Read the model definition and answer for the solid it produces. Units are mm, in the model's axes. A direction names the side the tool comes from. Coordinates: 2 decimals unless noted, no trailing zeros. Loops run counter-clockwise (first coordinate to the right, second up) from the corner with the lowest first, then second, coordinate; pieces in that order, holes last. Notation, with made-up numbers: (78, 64.25) - (124, 64.25) arc R17 cw to (124, 82.25) - close; hole circle Ø5 at (12, 61.25). An arc over 180 degrees is marked (long way). Use one line per item in the form item = value.
from build123d import *

# Parameters (mm, degrees)
SKETCH1_W                      = 75
SKETCH1_H                      = 54.33
BOSS_EXTRUDE1_DEPTH            = 45
CBORE_FOR_M4_SHCS1_D           = 4.5
CBORE_FOR_M4_SHCS1_CBORE_D     = 8
CBORE_FOR_M4_SHCS1_CBORE_DEPTH = 4
SKETCH4_OUTSIDE_W              = 97.592
SKETCH4_OUTSIDE_H              = 67.592
SKETCH4_OUTSIDE_W_2            = 75
SKETCH4_OUTSIDE_H_2            = 40
CUT_EXTRUDE1_DEPTH             = 55.33
SKETCH5_R                      = 8.5
CUT_EXTRUDE2_DEPTH             = 30
SKETCH5_3_R                    = 9
CUT_EXTRUDE3_DEPTH             = 20
SKETCH5_4_R                    = 11
CUT_EXTRUDE4_DEPTH             = 17
SKETCH6_R                      = 3.5
CUT_EXTRUDE5_DEPTH             = 55.33
SKETCH29_OUTSIDE_W             = 97.176
SKETCH29_OUTSIDE_H             = 76.506
SKETCH29_OUTSIDE_R             = 27.165
CUT_EXTRUDE6_DEPTH             = 34
SKETCH30_R                     = 4.5
CUT_EXTRUDE7_DEPTH             = 5


with BuildPart() as part:
    # Sketch1 → Boss-Extrude1 (new body)
    with BuildSketch(Plane.XY):
        Rectangle(SKETCH1_W, SKETCH1_H)
    extrude(amount=BOSS_EXTRUDE1_DEPTH)

    # CBORE for M4 SHCS1 (through all)
    with Locations(Plane.XY.offset(45)):
        with Locations((26.685, -23.265), (26.685, 23.265), (-26.685, 23.265), (-26.685, -23.265)):
            CounterBoreHole(CBORE_FOR_M4_SHCS1_D / 2, CBORE_FOR_M4_SHCS1_CBORE_D / 2, CBORE_FOR_M4_SHCS1_CBORE_DEPTH)

    # Sketch4 outside → Cut-Extrude1 (cut, through all)
    with BuildSketch(Plane.XZ.offset(27.165)):
        with Locations((0, 22.5)):
            Rectangle(SKETCH4_OUTSIDE_W, SKETCH4_OUTSIDE_H)
        with Locations((0, 20)):
            Rectangle(SKETCH4_OUTSIDE_W_2, SKETCH4_OUTSIDE_H_2, mode=Mode.SUBTRACT)
    extrude(amount=-CUT_EXTRUDE1_DEPTH, mode=Mode.SUBTRACT)

    # Sketch5 → Cut-Extrude2 (cut)
    with BuildSketch(Plane.XY.offset(40)):
        Circle(SKETCH5_R)
    extrude(amount=-CUT_EXTRUDE2_DEPTH, mode=Mode.SUBTRACT)

    # Sketch5<3> → Cut-Extrude3 (cut)
    with BuildSketch(Plane.XY.offset(40)):
        Circle(SKETCH5_3_R)
    extrude(amount=-CUT_EXTRUDE3_DEPTH, mode=Mode.SUBTRACT)

    # Sketch5<4> → Cut-Extrude4 (cut)
    with BuildSketch(Plane.XY.offset(40)):
        Circle(SKETCH5_4_R)
    extrude(amount=-CUT_EXTRUDE4_DEPTH, mode=Mode.SUBTRACT)

    # Sketch6 → Cut-Extrude5 (cut, through all)
    with BuildSketch(Plane(origin=(0, 27.165, 0), x_dir=(1, 0, 0), z_dir=(0, 1, 0))):
        with Locations((0, -30)):
            Circle(SKETCH6_R)
    extrude(amount=-CUT_EXTRUDE5_DEPTH, mode=Mode.SUBTRACT)

    # Sketch29 outside → Cut-Extrude6 (cut)
    with BuildSketch(Plane.XY.offset(40)):
        Rectangle(SKETCH29_OUTSIDE_W, SKETCH29_OUTSIDE_H)
        Circle(SKETCH29_OUTSIDE_R, mode=Mode.SUBTRACT)
    extrude(amount=-CUT_EXTRUDE6_DEPTH, mode=Mode.SUBTRACT)

    # Sketch30 → Cut-Extrude7 (cut)
    with BuildSketch(Plane(origin=(0, 0, 0), x_dir=(-1, 0, 0), z_dir=(0, 0, -1))):
        with Locations((-13.555, 11.3)):
            Circle(SKETCH30_R)
        with Locations((13.555, 11.3)):
            Circle(SKETCH30_R)
        with Locations((13.555, -11.3)):
            Circle(SKETCH30_R)
        with Locations((-13.555, -11.3)):
            Circle(SKETCH30_R)
    extrude(amount=-CUT_EXTRUDE7_DEPTH, mode=Mode.SUBTRACT)


solid = part.part
Item 1: Each of these flat-tipped pins is pushed along its axis until it touches: P1, Ø8, axis at x = -6.5, z = 26, coming from the -Y side; P2, Ø5, axis at x = -26.685, y = -23.265, coming from the +Z side; P3, Ø5, axis at y = 19, z = 33.5, coming from the -X side. Where does it stop, or does it pass through?
Results below:
P1 = -27.05
P2 = 6
P3 = -21.58
Item 2: Which of the six approach directions +Z, -Z, +X, -X, +Y, -Y give full straight-line access (tool end or side, diameter ignored) to faces 1 (the flat face through (37.5, 0, 3)), 2 (the flat face through (-27.35, 0.38, 6)), 3 (the flat face through (14, -11, 5)), 4 (the flat face through (0, 0, 10)), 5 (the flat face through (12, 0, 40))?
Results below:
face_1 = +Z, -Z, +X, +Y, -Y
face_2 = +Z, -X
face_3 = -Z
face_4 = +Z
face_5 = +Z, +X, -X, +Y, -Y
Item 3: The part is cut by section B-B on y = 0. Give the vertices of the cut face in (x, z) (3 decimals).
Results below:
outline = (-37.5, 0) - (37.5, 0) - (37.5, 6) - (27.165, 6) - (27.165, 40) - (11, 40) - (11, 23) - (9, 23) - (9, 20) - (8.5, 20) - (8.5, 10) - (-8.5, 10) - (-8.5, 20) - (-9, 20) - (-9, 23) - (-11, 23) - (-11, 40) - (-27.165, 40) - (-27.165, 6) - (-37.5, 6) - close
Item 4: For a pull along Z with two mould halves and no side action, classify faces 6 (the cylindrical face through (-0.46, -18.68, 26.53)), 7 (the flat face through (-1, 0, 0)), 8 (the flat face through (-1, -27.165, 3)) as +Z half, -Z half, draft (parallel to the pull), parting line (faces both ways), or undercut.
Results below:
face_6 = undercut
face_7 = -Z half
face_8 = draft
Item 5: Find the intervals of material crossed by L1, parallel to Z at x = 0, y = 22.5; L2, parallel to Y at x = -25, z = 5 (3 decimals); L3, parallel to Z at x = 22.5, y = 15.5, in increasing order.
Results below:
L1 = 0 to 26.5, 33.5 to 40
L2 = -27.165 to -24.756, -21.774 to 21.774, 24.756 to 27.165
L3 = 0 to 6
Item 6: The part is cut by section D-D on z = 36.5. Give the vertices of the cut face in (x, y) (3 decimals), plus the area to 3 significant figures.
Results below:
outline = circle Ø54.33 at (0, 0); hole circle Ø22 at (0, 0)
area = 1,940 mm²
Item 7: The part is cut by section C-C on x = -19. Give the vertices of the cut face in (y, z) (3 decimals), plus the area to 3 significant figures.
Results below:
outline = (-27.165, 0) - (27.165, 0) - (27.165, 6) - (19.415, 6) - (19.415, 40) - (-19.415, 40) - (-19.415, 6) - (-27.165, 6) - close
area = 1,650 mm²
Item 8: The part is cut by section A-A on z = 30. Give the vertices of the cut face in (x, y) (3 decimals), plus the area to 3 significant figures.
Results below:
outline = (-3.5, -26.939) - (-3.5, -10.428) arc R11 cw to (-3.5, 10.428) - (-3.5, 26.939) arc R27.165 ccw to start; (3.5, -26.939) arc R27.165 ccw to (3.5, 26.939) - (3.5, 10.428) arc R11 cw to (3.5, -10.428) - close
area = 1,710 mm²
